Geometry check sheet. Reference: the model listing, model coordinates, mm. Face numbers are marked on the shaded views. A direction names the side the tool comes from. Round coordinates to 2 decimals unless told otherwise and drop trailing zeros. Order: outer loops, then holes, each group sorted by start corner. A loop starts at its lowest first (then second) coordinate and runs counter-clockwise, first axis right, second up.
(1) Sectioned sample at B-B (z = 2.4). Record the boundary of the cut face in (x, y), plus the area to 3 significant figures.
(2) Set-up check for the marked faces 5 and 6: record each of +Z, -Z, +X, -X, +Y, -Y from which the full face is reachable in a straight line by a thin tool's end or side.
(3) Sectioned sample at C-C (y = 22.5). Record the boundary of the cut face in (x, z).
(4) Release check for a two-part mould opening along Y. For the marked faces 1, 2, 3 and 4 record: +Y half, -Y half, draft (parallel to the pull), parting line (faces both ways), or undercut.
(5) Go/stop test with flat-tipped pins: pin 1 (2.5 mm diameter, centred on x = 9, z = 1.5, fed in from +Y); pin 2 (3 mm diameter, centred on x = 5, y = 10.5, fed in from -Z). Record where each tip stops, or that it passes through.
(6) Material ranges on line 1 along X through (y, z) = (21, 3.1); line 2 along Y through (x, z) = (8, 3.35); line 3 along X through (y, z) = (47, 3.8), recorded low to high.
(7) Sectioned sample at A-A (x = 9). Record the boundary of the cut face in (y, z).
from build123d import *

# Parameters (mm, degrees)
BOSS_EXTRUDE1_DEPTH = 4.7752
SKETCH2_W           = 4.7752
SKETCH2_H           = 4.7752
CUT_EXTRUDE1_DEPTH  = 4.7752


with BuildPart() as part:
    # Sketch1 → Boss-Extrude1 (new body)
    with BuildSketch(Plane.XY):
        with BuildLine():
            Line((-4.5504, 44.7752), (-4.5504, 0.2248))
            ThreePointArc((-4.5504, 0.2248), (-3.085933906, -3.310733906), (0.4496, -4.7752))
            Line((0.4496, -4.7752), (7.4496, -4.7752))
            ThreePointArc((7.4496, -4.7752), (10.985133906, -3.310733906), (12.4496, 0.2248))
            Line((12.4496, 0.2248), (12.4496, 44.7752))
            ThreePointArc((12.4496, 44.7752), (10.985133906, 48.310733906), (7.4496, 49.7752))
            Line((7.4496, 49.7752), (0.4496, 49.7752))
            ThreePointArc((0.4496, 49.7752), (-3.085933906, 48.310733906), (-4.5504, 44.7752))
        make_face()
    extrude(amount=BOSS_EXTRUDE1_DEPTH)

    # Sketch2 → Cut-Extrude1 (cut)
    with BuildSketch(Plane(origin=(0, 0, 0), x_dir=(-1, 0, 0), z_dir=(0, 0, -1))):
        with Locations((-10.062, 22.5)):
            Rectangle(SKETCH2_W, SKETCH2_H)
    extrude(amount=-CUT_EXTRUDE1_DEPTH, mode=Mode.SUBTRACT)


solid = part.part
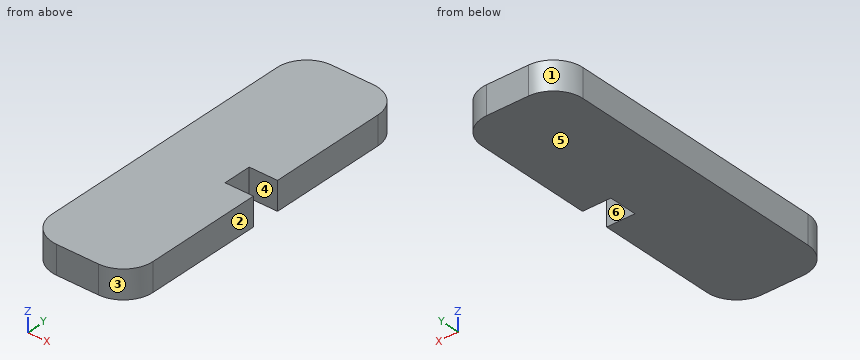
Answer below:
1. outline: (-4.55, 0.22) arc R5 ccw to (0.45, -4.78) - (7.45, -4.78) arc R5 ccw to (12.45, 0.22) - (12.45, 20.11) - (7.67, 20.11) - (7.67, 24.89) - (12.45, 24.89) - (12.45, 44.78) arc R5 ccw to (7.45, 49.78) - (0.45, 49.78) arc R5 ccw to (-4.55, 44.78) - close
1. area: 883 mm2
2. face 5: -Z, +X, -X, +Y, -Y
2. face 6: +Z, -Z, +X
3. outline: (-4.55, 0) - (7.67, 0) - (7.67, 4.78) - (-4.55, 4.78) - close
4. face 1: +Y half
4. face 2: draft
4. face 3: -Y half
4. face 4: undercut
5. pin 1: stops at y = 49.77
5. pin 2: stops at z = 0
6. line 1: x = -4.55 to 7.67
6. line 2: y = -4.74 to 20.11, 24.89 to 49.74
6. line 3: x = -4.03 to 11.93
7. outline: (-4.53, 0) - (20.11, 0) - (20.11, 4.78) - (-4.53, 4.78) - close; (24.89, 0) - (49.53, 0) - (49.53, 4.78) - (24.89, 4.78) - close
